Could you check a few things on this model? Use its own coordinates, in mm. Face numbers are marked on the shaded views. A direction names the side the tool comes from. Round coordinates to 2 decimals unless told otherwise and drop trailing zeros. Write each loop counter-clockwise with the first axis right and the second up, starting at its lowest first coordinate (ties: lowest second). Pieces come first, ordered by that corner, then holes. Notation, with made-up numbers: (-25.75, -16.5) - (-1.75, -16.5) arc R25 cw to (-1.75, 5.5) - close; hole circle Ø7 at (-15, 20.25). An arc over 180 degrees is marked (long way). Write each question's results on one line, items separated by ' | '. Start each with the question number.
(1) Imagine slicing it at D-D on z = -3. Write out the boundary of the cut face in (x, y) (3 decimals).
(2) Imagine slicing it at A-A on x = 0. Write out the boundary of the cut face in (y, z) (1 decimal).
(3) Imagine slicing it at C-C on z = 13. Write out the boundary of the cut face in (x, y), then the cut area to 3 significant figures.
(4) For P1, Ø5, axis at x = -8, z = 0, coming from the -Y side; P2, Ø3, axis at y = 3, z = 13, coming from the -X side; P3, Ø8, axis at x = -9, y = 21, coming from the -Z side, each with a flat end and sliding along its axis, tell me the tip position at first contact or that it passes through.
(5) Please list where these lines run through material, in increasing order: line 1 (Z direction, x = 13.5, y = 24); line 2 (Y direction, x = -11.5, z = -8.5); line 3 (Y direction, x = -5, z = -12). Write a range as [from, to].
(6) On a 3-axis mill with a long thin cutter (end or side, diameter ignored), from which of +Z, -Z, +X, -X, +Y, -Y can I reach the whole of each face in a straight line? I mean the marked faces 1, 2 and 3. Say none if no direction works.
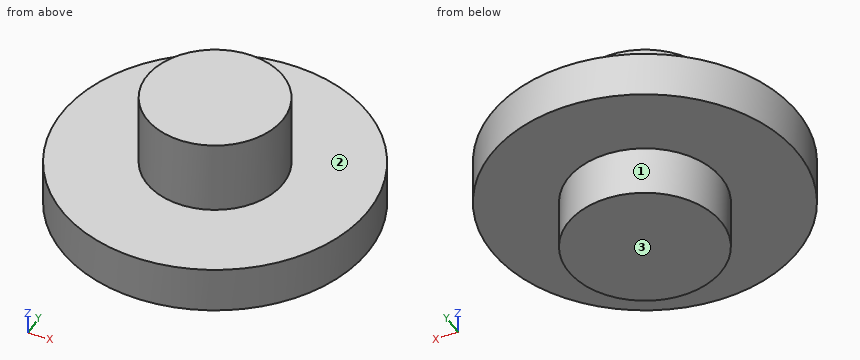
Autodesk Inventor part; units mm, degrees
ref_plane "YZ Plane" through (0, 0, 0) normal (1, 0, 0) x (0, 1, 0)
ref_plane "XZ Plane" through (0, 0, 0) normal (0, 1, 0) x (-1, 0, 0)
ref_plane "XY Plane" through (0, 0, 0) normal (0, 0, 1) x (1, 0, 0)
sketch "Sketch1" plane through (0, 0, 0) normal (0, 0, 1) x (1, 0, 0)
  circle A0 centre (0, 0) radius 28.575
  dimension "d0" = 57.15
extrude "Extrusion1" add sketch "Sketch1" along normal mid plane 8.636
sketch "Sketch2" plane through (0, 0, 4.318) normal (0, 0, 1) x (1, 0, 0)
  circle A0 centre (0, 0) radius 12.7
  dimension "d3" = 25.4
extrude "Extrusion2" add sketch "Sketch2" along normal blind 13.716
sketch "Sketch3" plane through (0, 0, -4.318) normal (0, 0, -1) x (-1, 0, 0)
  circle A0 centre (0, 0) radius 14.2875
  dimension "d6" = 28.575
extrude "Extrusion3" add sketch "Sketch3" along normal blind 9.4742
properties part number "newCoupler"
Response:
1) outline: circle Ø57.15 at (0, 0)
2) outline: (-28.6, -4.3) - (-14.3, -4.3) - (-14.3, -13.8) - (14.3, -13.8) - (14.3, -4.3) - (28.6, -4.3) - (28.6, 4.3) - (12.7, 4.3) - (12.7, 18) - (-12.7, 18) - (-12.7, 4.3) - (-28.6, 4.3) - close
3) outline: circle Ø25.4 at (0, 0) | area: 507 mm²
4) P1: y = -28.04 | P2: x = -12.61 | P3: z = -4.32
5) line 1: [-4.32, 4.32] | line 2: [-8.48, 8.48] | line 3: [-13.38, 13.38]
6) face 1: -Z | face 2: +Z | face 3: -Z, +X, -X, +Y, -Y
